Geometry check sheet. Reference: the model listing, model coordinates, mm. A direction names the side the tool comes from. Give positions to 0.01 mm unless a question says otherwise; leave off trailing zeros. Loops run counter-clockwise (first coordinate to the right, second up) from the corner with the lowest first, then second, coordinate; pieces in that order, holes last. Notation, with made-up numbers: (61.25, 20.25) -> (111.25, 20.25) arc R29 cw to (111.25, 40.25) -> close; hole circle Ø5 at (-4, 89.5). An arc over 180 degrees is marked (long way). One line per item, written item: value. Start each with the question number.
(1) Tool access check on faces 5 (the face through (10, 0, -12.5)), 6 (the face through (12.395, 6.021, -5.965)), 7 (the face through (10, 0, 12.5)), 8 (the face through (13, 1, -8.5)). Record the directions out of +Z, -Z, +X, -X, +Y, -Y that give a thin tool (end or side, any length) a straight path to the whole face; none if there is none.
(2) Scan lines: line 1 along X through (y, z) = (0.25, 10.25); line 2 along Y through (x, z) = (8.5, 10); line 3 along X through (y, z) = (0.75, -9.5). Record each from-to range of solid material in increasing order. Write a range as from..to.
(3) Sectioned sample at A-A, the plane x = 13.25. Record the cut outline in (y, z).
(4) Sectioned sample at C-C, the plane z = 0. Record the cut outline in (x, y), then the cut area to 3 significant figures.
(5) Draft check along X on faces 1 (the face through (10, 5.5, -13)), 2 (the face through (6.9, 1.57, 10.53)), 3 (the face through (14.9, 1.57, -10.47)), 4 (the face through (5, 4, 2)). Enter one of: pulls with the +X half, pulls with the -X half, needs draft (parallel to the pull), parting line crosses it, or undercut.
(6) Sectioned sample at D-D, the plane x = 8.5. Record the cut outline in (y, z).
(7) Gauge pin test, flat ends, axial feed: pin 1 Ø2 at (x, y) = (12.5, 1.5) entering from -Z; pin 2 Ø1.5 at (x, y) = (12.5, -1) entering from +Z; pin 3 Ø3 at (y, z) = (0.5, -3.5) entering from +X. Record the tip position at first contact, or that the pin passes through.
(8) Sectioned sample at B-B, the plane y = 1.5. Record the cut outline in (x, z).
from build123d import *

# Parameters (mm, degrees)
SKETCH_1_W          = 25
SKETCH_1_H          = 11
SKETCH_1_R          = 2.6
EXTRUDE_1_DEPTH     = 5
SKETCH_2_W          = 4
SKETCH_2_H          = 11
EXTRUDE_2_DEPTH     = 15
SKETCH_4_R          = 1.6
CUT_EXTRUDE_1_DEPTH = 33.484611742
EXTRUDE_4_DEPTH     = 2
EXTRUDE_3_DEPTH     = 3
SKETCH_8_W          = 20
SKETCH_8_H          = 25
CUT_EXTRUDE_2_DEPTH = 3


with BuildPart() as part:
    # 草图1 → 凸台-拉伸1 (new body)
    with BuildSketch(Plane(origin=(0, 0, 0), x_dir=(0, 0, -1), z_dir=(1, 0, 0))):
        Rectangle(SKETCH_1_W, SKETCH_1_H)
        with Locations((0, 1.5)):
            Circle(SKETCH_1_R, mode=Mode.SUBTRACT)
    extrude(amount=EXTRUDE_1_DEPTH)

    # 草图2 → 凸台-拉伸2 (add)
    with BuildSketch(Plane(origin=(5, 0, 0), x_dir=(0, 0, -1), z_dir=(1, 0, 0))):
        with Locations((-10.5, 0)):
            Rectangle(SKETCH_2_W, SKETCH_2_H)
        with Locations((10.5, 0)):
            Rectangle(SKETCH_2_W, SKETCH_2_H)
    extrude(amount=EXTRUDE_2_DEPTH)

    # 草图4 → 切除-拉伸1 (cut, through all)
    with BuildSketch(Plane.XY.offset(12.5)):
        with Locations((16.5, 1.5)):
            Circle(SKETCH_4_R)
        with Locations((8.5, 1.5)):
            Circle(SKETCH_4_R)
    extrude(amount=-CUT_EXTRUDE_1_DEPTH, mode=Mode.SUBTRACT)

    # 草图7 → 凸台-拉伸4 (add)
    with BuildSketch(Plane(origin=(0, 5.5, 0), x_dir=(1, 0, 0), z_dir=(0, 1, 0))):
        Polygon((20, 8.5), (5, 8.5), (5, -8.5), (20, -8.5), (20, -14), (0, -14), (0, -8.5), (0, 8.5), (0, 14), (20, 14), align=None)
    extrude(amount=EXTRUDE_4_DEPTH)

    # 草图6 → 凸台-拉伸3 (add)
    with BuildSketch(Plane.XZ.offset(-7.5)):
        Polygon((20, 8.5), (5, 8.5), (5, 3.5), align=None)
        Polygon((5, -8.5), (5, -3.5), (20, -8.5), align=None)
    extrude(amount=EXTRUDE_3_DEPTH)

    # 草图8 → 切除-拉伸2 (cut)
    with BuildSketch(Plane.XZ.offset(5.5)):
        with Locations((10, 0)):
            Rectangle(SKETCH_8_W, SKETCH_8_H)
    extrude(amount=-CUT_EXTRUDE_2_DEPTH, mode=Mode.SUBTRACT)


solid = part.part
Calculated:
1. face 5: -Z, +X, -X, -Y
1. face 6: +X, +Y, -Y
1. face 7: +Z, +X, -X, -Y
1. face 8: +X, -Y
2. line 1: x = 0..7.5, 9.5..15.5, 17.5..20
2. line 2: y = -2.5..-0.1, 3.1..7.5
2. line 3: x = 0..7.09, 9.91..15.09, 17.91..20
3. outline: (-2.5, -12.5) -> (5.5, -12.5) -> (5.5, -14) -> (7.5, -14) -> (7.5, -6.25) -> (4.5, -6.25) -> (4.5, -8.5) -> (-2.5, -8.5) -> close; (-2.5, 8.5) -> (4.5, 8.5) -> (4.5, 6.25) -> (7.5, 6.25) -> (7.5, 14) -> (5.5, 14) -> (5.5, 12.5) -> (-2.5, 12.5) -> close
4. outline: (0, -2.5) -> (5, -2.5) -> (5, -1.1) -> (0, -1.1) -> close; (0, 4.1) -> (5, 4.1) -> (5, 7.5) -> (0, 7.5) -> close
4. area: 24.0 mm2
5. face 1: needs draft
5. face 2: undercut
5. face 3: undercut
5. face 4: pulls with the +X half
6. outline: (-2.5, -12.5) -> (-0.1, -12.5) -> (-0.1, -8.5) -> (-2.5, -8.5) -> close; (-2.5, 8.5) -> (-0.1, 8.5) -> (-0.1, 12.5) -> (-2.5, 12.5) -> close; (3.1, -12.5) -> (5.5, -12.5) -> (5.5, -14) -> (7.5, -14) -> (7.5, -4.67) -> (4.5, -4.67) -> (4.5, -8.5) -> (3.1, -8.5) -> close; (3.1, 8.5) -> (4.5, 8.5) -> (4.5, 4.67) -> (7.5, 4.67) -> (7.5, 14) -> (5.5, 14) -> (5.5, 12.5) -> (3.1, 12.5) -> close
7. pin 1: stops at z = -12.5
7. pin 2: stops at z = 12.5
7. pin 3: stops at x = 5
8. outline: (0, -12.5) -> (6.9, -12.5) -> (6.9, -8.5) -> (5, -8.5) -> (5, -2.6) -> (0, -2.6) -> close; (0, 2.6) -> (5, 2.6) -> (5, 8.5) -> (6.9, 8.5) -> (6.9, 12.5) -> (0, 12.5) -> close; (10.1, -12.5) -> (14.9, -12.5) -> (14.9, -8.5) -> (10.1, -8.5) -> close; (10.1, 8.5) -> (14.9, 8.5) -> (14.9, 12.5) -> (10.1, 12.5) -> close; (18.1, -12.5) -> (20, -12.5) -> (20, -8.5) -> (18.1, -8.5) -> close; (18.1, 8.5) -> (20, 8.5) -> (20, 12.5) -> (18.1, 12.5) -> close
